Read the model definition and answer for the solid it produces. Units are mm, in the model's axes. Face numbers are marked on the shaded views. Coordinates: 2 decimals unless noted, no trailing zeros. Order: outer loops, then holes, each group sorted by start corner. A loop starts at its lowest first (then second) coordinate and runs counter-clockwise, first axis right, second up.
Autodesk Inventor part; units mm, degrees
ref_plane "YZ Plane" through (0, 0, 0) normal (1, 0, 0) x (0, 1, 0)
ref_plane "XZ Plane" through (0, 0, 0) normal (0, 1, 0) x (-1, 0, 0)
ref_plane "XY Plane" through (0, 0, 0) normal (0, 0, 1) x (1, 0, 0)
sketch "Sketch1" plane through (0, 0, 0) normal (0, 1, 0) x (-1, 0, 0)
  line L0 (0, 0) -> (-6, 0)
  line L1 (-6, 0) -> (-6, -20)
  line L2 (-6, -20) -> (0, -20)
  line L3 (0, -20) -> (0, 0)
  line L4 (0, 0) -> (-2.5, 0)
  line L5 (0, -10) -> (-2.5, -10)
  line L6 (-2.5, -8) -> (-2.5, 0)
  line L7 (0, -20) -> (-4, -20)
  line L8 (-4, -20) -> (-4, -11.1225)
  line L9 (-4, -10) -> (-4.5, -10)
  arc A0 (-3.25, -9.5612) -> (-2.5, -8) centre (-4.5, -8) ccw
  arc A1 (-3.25, -9.5612) -> (-4, -11.1225) centre (-2, -11.1225) ccw
  dimension "d0" = 6
  dimension "d1" = 20
  dimension "d2" = 2.5
  dimension "d3" = 4
  dimension "d4" = 2
revolve "Revolution1" add sketch "Sketch1" angle 360 about axis through (0, 0, -20) along (0, 0, 1) contours L6 A0 A1 L8 L2 L1 L0
ref_plane "Work Plane1" through (0, 0, -10) normal (0, 0, 1) x (1, 0, 0)
properties part number "motorCoupling5_8"
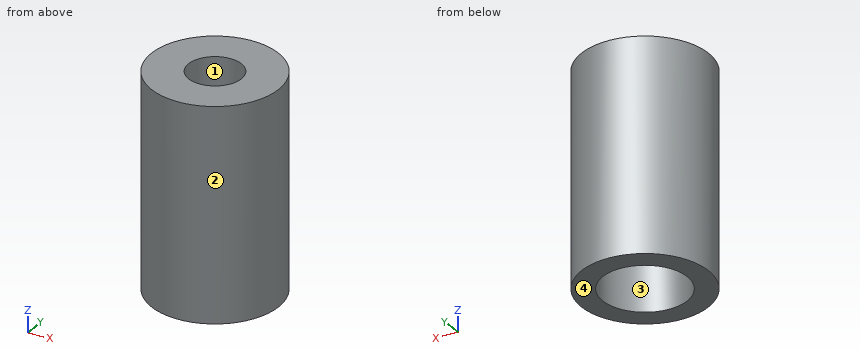
Q1. The part is cut by section A-A, the plane x = 0. Determine the outline of the cut face in (y, z).
Q2. Determine the mould class of the marked faces 1, 2, 3 and 4 for opening direction X: +X half, -X half, draft (parallel to the pull), parting line (faces both ways), or undercut.
Q3. Each of these flat-tipped pins is pushed along its axis until it touches: P1, Ø2, axis at y = 4.5, z = -17.5, coming from the -X side; P2, Ø4, axis at x = -2.5, z = -3.5, coming from the +Y side; P3, Ø3, axis at y = 4, z = -12, coming from the +X side; P4, Ø5, axis at y = 0.5, z = -16, coming from the -X side. Where does it stop, or does it pass through?
Q4. The part is cut by section D-D, the plane x = -5. Determine the outline of the cut face in (y, z).
Q5. Straight lines are drawn through the part: L1, parallel to Y at x = 0, z = -15.25; L2, parallel to Y at x = 0, z = -3.75; L3, parallel to X at y = 2, z = -18.5. For each, find the intervals that lie inside material, in ascending order.
Q6. The part is cut by section C-C, the plane z = -7.25. Determine the outline of the cut face in (x, y).
Computed values:
1. outline: (-6, -20) - (-4, -20) - (-4, -11.12) arc R2 cw to (-3.25, -9.56) arc R2 ccw to (-2.5, -8) - (-2.5, 0) - (-6, 0) - close; (2.5, -8) arc R2 ccw to (3.25, -9.56) arc R2 cw to (4, -11.12) - (4, -20) - (6, -20) - (6, 0) - (2.5, 0) - close
2. face 1: undercut
2. face 2: parting line
2. face 3: undercut
2. face 4: draft
3. P1: stops at x = -4.87
3. P2: stops at y = 5.98
3. P3: stops at x = 5.45
3. P4: stops at x = -6
4. outline: (-3.32, -20) - (3.32, -20) - (3.32, 0) - (-3.32, 0) - close
5. L1: y = -6 to -4, 4 to 6
5. L2: y = -6 to -2.5, 2.5 to 6
5. L3: x = -5.66 to -3.46, 3.46 to 5.66
6. outline: circle Ø12 at (0, 0); hole circle Ø5 at (0, 0)
